For this review, take the finished solid that the model builds, in its own axes (mm). Round coordinates to 2 decimals unless told otherwise and drop trailing zeros. Write each loop counter-clockwise with the first axis right and the second up, starting at its lowest first coordinate (ties: lowest second). Pieces come first, ordered by that corner, then holes. Notation, with made-up numbers: M 69,44.5 L 98,44.5 A23 cw 98,53.5 Z; hole C 11.25,-15.75 d3. An arc over 180 degrees is marked long. Use one line per item in the form item = value. Start each with the question number.
Item 1: Add section A-A (z = 90). State the section outline as (x, y) points.
Item 2: Add section B-B (x = 115). State the section outline as (y, z) points.
Item 3: Add section D-D (z = 64.5). State the section outline as (x, y) points.
Item 4: For line 1 (Z direction, x = 422.5, y = -14.75); line 2 (Z direction, x = 24.5, y = -10); line 3 (Z direction, x = 335, y = -2.5), list the stretches that pass through material, from the lowest coordinate up. Write a range as [from, to].
Item 5: Add section C-C (x = 335). State the section outline as (y, z) points, and give its area (3 significant figures).
Item 6: For P1, Ø4, axis at y = -8, z = 22, coming from the +X side; P2, Ø7.5, axis at x = 199.5, z = 91, coming from the -Y side; P3, Ø4, axis at y = -2, z = 29, coming from the -X side, all flat-tipped, find the tip position at first contact; note any pin that passes through.
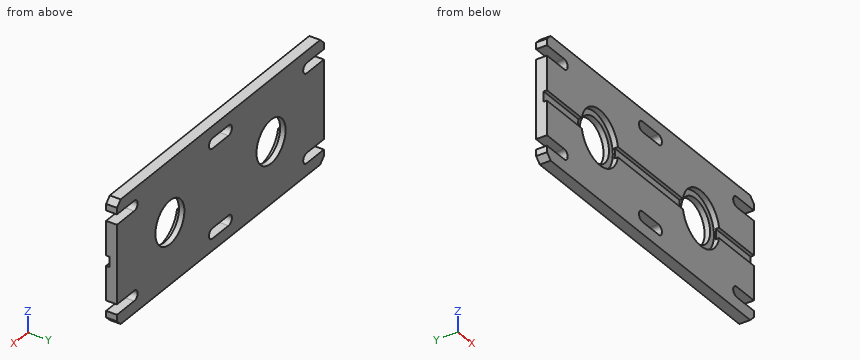
from build123d import *

# Parameters (mm, degrees)
F0_W      = 450
F0_H      = 180
F1_DEPTH  = 16
F2_SIZE   = 8
F3_R      = 31.6
F3_R_2    = 31.65
F4_DEPTH  = 16.001
F6_DEPTH  = 16.001
F7_R      = 40
F7_R_2    = 31.65
F8_DEPTH  = 8
F9_R      = 40
F10_DEPTH = 8
F11_W     = 10
F11_H     = 15
F12_DEPTH = 450.001


with BuildPart() as f1:
    # F0 (on Front) → F1 (new body)
    with BuildSketch(Plane.XZ):
        with Locations((225, 90)):
            Rectangle(F0_W, F0_H)
    extrude(amount=F1_DEPTH)

    # F2
    f2_edges = [f1.edges().sort_by_distance(p)[0] for p in [
        (450, -8, 180),
        (450, -8, 0),
        (0, -8, 180),
        (0, -8, 0),
    ]]
    chamfer(f2_edges, length=F2_SIZE)

    # F3 (on face) → F4 (cut, through all)
    with BuildSketch(Plane.XZ.offset(16)):
        with Locations((335, 90)):
            Circle(F3_R)
        with Locations((115, 90)):
            Circle(F3_R_2)
    extrude(amount=-F4_DEPTH, mode=Mode.SUBTRACT)

    # F5 (on face) → F6 (cut, through all)
    with BuildSketch(Plane.XZ.offset(16)):
        with BuildLine():
            Line((207.5, 147.5), (242.5, 147.5))
            ThreePointArc((242.5, 147.5), (247.803301, 149.696699), (250, 155))
            ThreePointArc((250, 155), (247.803301, 160.303301), (242.5, 162.5))
            Line((242.5, 162.5), (207.5, 162.5))
            ThreePointArc((207.5, 162.5), (202.196699, 160.303301), (200, 155))
            ThreePointArc((200, 155), (202.196699, 149.696699), (207.5, 147.5))
        make_face()
        with BuildLine():
            Line((-68.917155, 147.5), (37.5, 147.5))
            ThreePointArc((37.5, 147.5), (42.803301, 149.696699), (45, 155))
            ThreePointArc((45, 155), (42.803301, 160.303301), (37.5, 162.5))
            Line((37.5, 162.5), (-68.917155, 162.5))
            Line((-68.917155, 162.5), (-68.917155, 147.5))
        make_face()
        with BuildLine():
            Line((455.818099, 147.5), (455.818099, 162.5))
            Line((455.818099, 162.5), (412.5, 162.5))
            ThreePointArc((412.5, 162.5), (407.196699, 160.303301), (405, 155))
            ThreePointArc((405, 155), (407.196699, 149.696699), (412.5, 147.5))
            Line((412.5, 147.5), (455.818099, 147.5))
        make_face()
        with BuildLine():
            ThreePointArc((207.5, 32.5), (202.196699, 30.303301), (200, 25))
            ThreePointArc((200, 25), (202.196699, 19.696699), (207.5, 17.5))
            Line((207.5, 17.5), (242.5, 17.5))
            ThreePointArc((242.5, 17.5), (247.803301, 19.696699), (250, 25))
            ThreePointArc((250, 25), (247.803301, 30.303301), (242.5, 32.5))
            Line((242.5, 32.5), (207.5, 32.5))
        make_face()
        with BuildLine():
            ThreePointArc((412.5, 32.5), (407.196699, 30.303301), (405, 25))
            ThreePointArc((405, 25), (407.196699, 19.696699), (412.5, 17.5))
            Line((412.5, 17.5), (455.818099, 17.5))
            Line((455.818099, 17.5), (455.818099, 32.5))
            Line((455.818099, 32.5), (412.5, 32.5))
        make_face()
        with BuildLine():
            ThreePointArc((37.5, 17.5), (42.803301, 19.696699), (45, 25))
            ThreePointArc((45, 25), (42.803301, 30.303301), (37.5, 32.5))
            Line((37.5, 32.5), (-68.917155, 32.5))
            Line((-68.917155, 32.5), (-68.917155, 17.5))
            Line((-68.917155, 17.5), (37.5, 17.5))
        make_face()
    extrude(amount=-F6_DEPTH, mode=Mode.SUBTRACT)

    # F7 (on face) → F8 (cut)
    with BuildSketch(Plane.XZ.offset(16)):
        with Locations((115, 90)):
            Circle(F7_R)
        with Locations((115, 90)):
            Circle(F7_R_2, mode=Mode.SUBTRACT)
    extrude(amount=-F8_DEPTH, mode=Mode.SUBTRACT)

    # F9 (on face) → F10 (cut)
    with BuildSketch(Plane.XZ.offset(16)):
        with Locations((335, 90)):
            Circle(F9_R)
    extrude(amount=-F10_DEPTH, mode=Mode.SUBTRACT)

    # F11 (on face) → F12 (cut, through all)
    with BuildSketch(Plane(origin=(0, 0, 0), x_dir=(0, -1, 0), z_dir=(-1, 0, 0))):
        with Locations((16, 90)):
            Rectangle(F11_W, F11_H)
    extrude(amount=-F12_DEPTH, mode=Mode.SUBTRACT)


solid = f1.part
Calculated:
q1.outline = M 0,-11 L 75,-11 L 75,-8 L 83.35,-8 L 83.35,0 L 0,0 Z; M 146.65,-8 L 155,-8 L 155,-11 L 295,-11 L 295,-8 L 303.4,-8 L 303.4,0 L 146.65,0 Z; M 366.6,-8 L 375,-8 L 375,-11 L 450,-11 L 450,0 L 366.6,0 Z
q2.outline = M -16,0 L 0,0 L 0,58.35 L -8,58.35 L -8,50 L -16,50 Z; M -16,130 L -8,130 L -8,121.65 L 0,121.65 L 0,180 L -16,180 Z
q3.outline = M 0,-16 L 84.18,-16 L 84.18,-8 L 96.25,-8 L 96.25,0 L 0,0 Z; M 133.75,-8 L 145.82,-8 L 145.82,-16 L 304.18,-16 L 304.18,-8 L 316.34,-8 L 316.34,0 L 133.75,0 Z; M 353.66,-8 L 365.82,-8 L 365.82,-16 L 450,-16 L 450,0 L 353.66,0 Z
q4.line_1 = [0, 17.5], [32.5, 82.5], [97.5, 147.5], [162.5, 180]
q4.line_2 = [0, 17.5], [32.5, 147.5], [162.5, 180]
q4.line_3 = [0, 58.4], [121.6, 180]
q5.outline = M -16,0 L 0,0 L 0,58.4 L -8,58.4 L -8,50 L -16,50 Z; M -16,130 L -8,130 L -8,121.6 L 0,121.6 L 0,180 L -16,180 Z
q5.area = 1,730 mm^2
q6.P1 = 406.91
q6.P2 = -11
q6.P3 = 42
